from build123d import *

# Parameters (mm, degrees)
F0_W     = 138.64535
F0_H     = 54.796886
F1_DEPTH = 25.4
F3_D     = 76.2
F5_D     = 14.2748


with BuildPart() as f1:
    # F0 (on Front) → F1 (new body)
    with BuildSketch(Plane.XZ):
        with Locations((0, -27.398443)):
            Rectangle(F0_W, F0_H)
    extrude(amount=F1_DEPTH)

    # F3 (through all)
    with Locations(Plane.XZ.offset(25.4)):
        with Locations((0, 0)):
            Hole(F3_D / 2)

    # F5 (through all)
    with Locations(Plane.XY):
        with Locations((53.711338, -12.7), (-52.589513, -12.598515)):
            Hole(F5_D / 2)


solid = f1.part
Source: CAD feature listing. Evaluate the final solid. Frame: model axes, mm. Round coordinates to 2 decimals unless told otherwise and drop trailing zeros. Loops run counter-clockwise (first coordinate to the right, second up) from the corner with the lowest first, then second, coordinate; pieces in that order, holes last. Notation, with made-up numbers: M -11,85.25 L 26,85.25 A36 cw 26,119.25 Z; hole C 82.25,14.25 d11. An arc over 180 degrees is marked long. Return JSON: item names as keys, results as strings. Group by question number.
1. Pin query (flat end, axial travel): pin 1 (13 mm diameter, centred on x = 53.71, y = -12.7, fed in from +Z). Return the tip coordinate at first contact, or that it passes through.
2. Material intervals for line 1 along X through (y, z) = (-12.5, -46.5); line 2 along X through (y, z) = (-8.75, -24); line 3 along X through (y, z) = (-9.25, -10.5), sorted ascending. Write a range as from..to.
3. Section query D-D on z = -26. Output: boundary loops of the cut face in (x, y), and give its area (3 significant figures).
4. Section query B-B on x = -56.5. Output: boundary loops of the cut face in (y, z).
5. Mould query, pull axis Y, two halves, no side actions, for faces 1 (the face through (-1, 0, -39)), 2 (the face through (-57.4, -18.2, 0)), 3 (the face through (60.842, -12.386, -27.782)). Classes: released by +Y, released by -Y, zero draft, split by the parting line, or undercut.
6. Section query C-C on y = -23.5. Output: boundary loops of the cut face in (x, z).
7. Section query A-A on z = -13.5. Output: boundary loops of the cut face in (x, y).
Checks:
{
 "1": {"pin 1": "passes through"},
 "2": {"line 1": "x = -69.32..-59.73, -45.45..46.58, 60.85..69.32", "line 2": "x = -69.32..-58.6, -46.58..-29.59, 29.59..47.77, 59.66..69.32", "line 3": "x = -69.32..-58.89, -46.29..-36.62, 36.62..47.46, 59.96..69.32"},
 "3": {"outline": "M -69.32,-25.4 L -27.85,-25.4 L -27.85,0 L -69.32,0 Z; M 27.85,-25.4 L 69.32,-25.4 L 69.32,0 L 27.85,0 Z; hole C -52.59,-12.6 d14.27; hole C 53.71,-12.7 d14.27", "area": "1,790 mm²"},
 "4": {"outline": "M -25.4,-54.8 L -18.57,-54.8 L -18.57,0 L -25.4,0 Z; M -6.63,-54.8 L 0,-54.8 L 0,0 L -6.63,0 Z"},
 "5": {"face 1": "released by +Y", "face 2": "zero draft", "face 3": "undercut"},
 "6": {"outline": "M -69.32,-54.8 L 69.32,-54.8 L 69.32,0 L 38.1,0 A38.1 cw -38.1,0 L -69.32,0 Z"},
 "7": {"outline": "M -69.32,-25.4 L -35.63,-25.4 L -35.63,0 L -69.32,0 Z; M 35.63,-25.4 L 69.32,-25.4 L 69.32,0 L 35.63,0 Z; hole C -52.59,-12.6 d14.27; hole C 53.71,-12.7 d14.27"}
}
